```python
from build123d import *

# Parameters (mm, degrees)
F0_R     = 10
F0_R_2   = 4.25
F1_DEPTH = 10
F3_DEPTH = 53
F5_DEPTH = 25
F6_DEPTH = 23
F7_R     = 9.99999
F8_D     = 8.5


# Not quite as in the source:
# - a fillet or chamfer is up to 0.001 mm smaller than in the source, because OpenCascade refuses the exact size
# - a feature names something its author has since deleted; it is built from what else it names


with BuildPart() as f1:
    # F0 (on Top) → F1 (new body)
    with BuildSketch(Plane.XY):
        Circle(F0_R)
        Circle(F0_R_2, mode=Mode.SUBTRACT)
    extrude(amount=F1_DEPTH)

    # F2 (on face) → F3 (join)
    with BuildSketch(Plane.XY):
        with BuildLine():
            ThreePointArc((8.6602540378, -5), (5, -8.6602540378), (0, -10))
            Line((0, -10), (10, -10))
            Line((10, -10), (10, -5))
            Line((10, -5), (8.6602540378, -5))
        make_face()
        with BuildLine():
            ThreePointArc((-8.6602540378, -5), (-5, -8.6602540378), (0, -10))
            ThreePointArc((0, -10), (5, -8.6602540378), (8.6602540378, -5))
            Line((8.6602540378, -5), (-8.6602540378, -5))
        make_face()
        with BuildLine():
            Line((-10, -10), (0, -10))
            ThreePointArc((0, -10), (-5, -8.6602540378), (-8.6602540378, -5))
            Line((-8.6602540378, -5), (-10, -5))
            Line((-10, -5), (-10, -10))
        make_face()
        with BuildLine():
            Line((8.6602540378, 5), (10, 5))
            Line((10, 5), (10, 10))
            Line((10, 10), (-2.67e-08, 10))
            ThreePointArc((-2.67e-08, 10), (4.9999999884, 8.6602540445), (8.6602540378, 5))
        make_face()
        with BuildLine():
            Line((-10, 10), (-10, 5))
            Line((-10, 5), (-8.6602540378, 5))
            ThreePointArc((-8.6602540378, 5), (-5.0000000116, 8.6602540312), (-2.67e-08, 10))
            Line((-2.67e-08, 10), (-10, 10))
        make_face()
        with BuildLine():
            ThreePointArc((-2.67e-08, 10), (-5.0000000116, 8.6602540312), (-8.6602540378, 5))
            Line((-8.6602540378, 5), (8.6602540378, 5))
            ThreePointArc((8.6602540378, 5), (4.9999999884, 8.6602540445), (-2.67e-08, 10))
        make_face()
    extrude(amount=-F3_DEPTH)

    # F4 (on face) → F5 (cut)
    with BuildSketch(Plane.XZ.offset(10)):
        with BuildLine():
            ThreePointArc((2.5, -43), (-1.767766953, -41.232233047), (0, -45.5))
            ThreePointArc((0, -45.5), (1.767766953, -44.767766953), (2.5, -43))
        make_face()
    extrude(amount=-F5_DEPTH, mode=Mode.SUBTRACT)

    # F2 (on face) → F6 (join)
    with BuildSketch(Plane.XY):
        with BuildLine():
            ThreePointArc((4.25, 0), (0, 4.25), (-4.25, 0))
            Line((-4.25, 0), (4.25, 0))
        make_face()
        with BuildLine():
            ThreePointArc((-10, 0), (-9.6592582629, -2.588190451), (-8.6602540378, -5))
            Line((-8.6602540378, -5), (8.6602540378, -5))
            ThreePointArc((8.6602540378, -5), (9.6592582629, -2.588190451), (10, 0))
            Line((10, 0), (4.25, 0))
            ThreePointArc((4.25, 0), (0, -4.25), (-4.25, 0))
            Line((-4.25, 0), (-10, 0))
        make_face()
        with BuildLine():
            ThreePointArc((-8.6602540378, 5), (-9.6592582629, 2.588190451), (-10, 0))
            Line((-10, 0), (-4.25, 0))
            ThreePointArc((-4.25, 0), (0, 4.25), (4.25, 0))
            Line((4.25, 0), (10, 0))
            ThreePointArc((10, 0), (9.6592582629, 2.588190451), (8.6602540378, 5))
            Line((8.6602540378, 5), (-8.6602540378, 5))
        make_face()
        with BuildLine():
            Line((-10, 5), (-10, 0))
            ThreePointArc((-10, 0), (-9.6592582629, 2.588190451), (-8.6602540378, 5))
            Line((-8.6602540378, 5), (-10, 5))
        make_face()
        with BuildLine():
            Line((-10, -5), (-8.6602540378, -5))
            ThreePointArc((-8.6602540378, -5), (-9.6592582629, -2.588190451), (-10, 0))
            Line((-10, 0), (-10, -5))
        make_face()
        with BuildLine():
            ThreePointArc((8.6602540378, 5), (9.6592582629, 2.588190451), (10, 0))
            Line((10, 0), (10, 5))
            Line((10, 5), (8.6602540378, 5))
        make_face()
        with BuildLine():
            ThreePointArc((10, 0), (9.6592582629, -2.588190451), (8.6602540378, -5))
            Line((8.6602540378, -5), (10, -5))
            Line((10, -5), (10, 0))
        make_face()
        with BuildLine():
            Line((4.25, 0), (-4.25, 0))
            ThreePointArc((-4.25, 0), (0, -4.25), (4.25, 0))
        make_face()
    extrude(amount=-F6_DEPTH)

    # F7 (radius 10 in the source; OpenCascade refuses exactly that, so slightly less here)
    f7_edges = [f1.edges().sort_by_distance(p)[0] for p in [
        (-10, -7.5, -53),
        (-10, 7.5, -53),
        (10, 7.5, -53),
        (10, -7.5, -53),
    ]]
    fillet(f7_edges, radius=F7_R)

    # F8 (through all)
    with Locations(Plane.XY):
        with Locations((0, 0)):
            Hole(F8_D / 2)


solid = f1.part
```
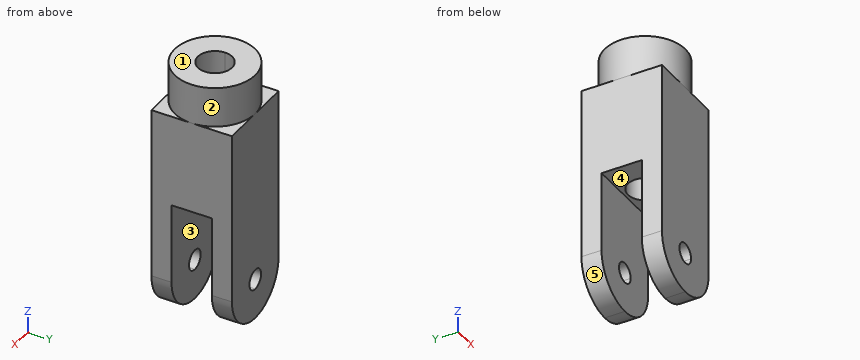
CAD build for the part. Positions are in the model's coordinates, mm. Face numbers are marked on the shaded views. A direction names the side the tool comes from. Coordinates: 2 decimals unless noted, no trailing zeros. Order: outer loops, then holes, each group sorted by start corner. A loop starts at its lowest first (then second) coordinate and runs counter-clockwise, first axis right, second up. Notation, with made-up numbers: (61.5, -38.5) -> (103.5, -38.5) arc R26 cw to (103.5, -20.5) -> close; hole circle Ø9 at (-3, -24.5). An arc over 180 degrees is marked (long way). Use one line per item in the form item = value. Start each with the question number.
1) Band-saw the part on D-D on x = -8. Give the cut face in (y, z), then the cut area to 3 significant figures.
2) Band-saw the part on B-B on z = -34.5. Give the cut face in (x, y).
3) Drop flat-ended pins along their axis: pin 1 (12 mm diameter, centred on y = 1, z = -24, fed in from -X); pin 2 (8 mm diameter, centred on x = 0.5, y = -0.5, fed in from -Z); pin 3 (1.5 mm diameter, centred on x = -7.5, y = 6, fed in from -Z). Give the stop position or say it passes through.
4) Band-saw the part on C-C on y = -3.5. Give the cut face in (x, z), then the cut area to 3 significant figures.
5) Tool access for the marked faces 4 and 5: list every direction of +Z, -Z, +X, -X, +Y, -Y with a clear straight run to the whole face (end or side of a thin tool).
6) Drill centre lines: L1, parallel to X at y = 6.7, z = -43; L2, parallel to Y at x = -7.5, z = -46; L3, parallel to Y at x = 0, z = -15.25. Where is each one in solid material? Low to high. Write a range as [from, to].
7) Pull direction Y, two halves, no side cores. Call the marked faces 1, 2 and 3: +Y half, -Y half, draft (parallel to the pull), parting line (faces both ways), or undercut.
8) Band-saw the part on A-A on z = -14.5. Give the cut face in (x, y).
Entries:
q1.outline = (-10, -49) -> (-5, -49) -> (-5, -23) -> (5, -23) -> (5, -49) -> (10, -49) -> (10, 0) -> (6, 0) -> (6, 10) -> (-6, 10) -> (-6, 0) -> (-10, 0) -> close
q1.area = 840 mm2
q2.outline = (-10, -10) -> (10, -10) -> (10, -5) -> (-10, -5) -> close; (-10, 5) -> (10, 5) -> (10, 10) -> (-10, 10) -> close
q3.pin_1 = -10
q3.pin_2 = -23
q3.pin_3 = -50.38
q4.outline = (-10, -23) -> (-2.41, -23) -> (-2.41, 10) -> (-9.37, 10) -> (-9.37, 0) -> (-10, 0) -> close; (2.41, -23) -> (10, -23) -> (10, 0) -> (9.37, 0) -> (9.37, 10) -> (2.41, 10) -> close
q4.area = 488 mm2
q5.face_4 = -Z, +X, -X
q5.face_5 = -Z, -X, +Y, -Y
q6.L1 = [-10, -2.5], [2.5, 10]
q6.L2 = [-10, -5], [5, 10]
q6.L3 = [-10, -4.25], [4.25, 10]
q7.face_1 = draft
q7.face_2 = parting line
q7.face_3 = undercut
q8.outline = (-10, -10) -> (10, -10) -> (10, 10) -> (-10, 10) -> close; hole circle Ø8.5 at (0, 0)
